Autodesk Inventor part; units mm, degrees
ref_plane "YZ Plane" through (0, 0, 0) normal (1, 0, 0) x (0, 1, 0)
ref_plane "XZ Plane" through (0, 0, 0) normal (0, 1, 0) x (-1, 0, 0)
ref_plane "XY Plane" through (0, 0, 0) normal (0, 0, 1) x (1, 0, 0)
sketch "スケッチ5" plane through (0, 0, 0) normal (1, 0, 0) x (0, 1, 0)
  line L0 (0, 0) -> (0, 1.2936) construction
  line L1 (0, 0) -> (-1.3338, 0) construction
  line L2 (2, 2) -> (-2, 2)
  line L3 (-2, 2) -> (-2, 0)
  line L4 (-2, 0) -> (2, 0)
  line L5 (2, 0) -> (2, 2)
  line L6 (0.8, 2) -> (0.8, 0)
  line L7 (-0.8, 2) -> (-0.8, 0)
  line L8 (-2, 1) -> (2, 1) construction
  line L9 (2, 1) -> (7.1642, 10.7124) construction
  line L10 (8.0471, 10.243) -> (6.2812, 11.1819)
  line L11 (6.2812, 11.1819) -> (0.7025, 0.6899)
  line L12 (0.7025, 0.6899) -> (2.4684, -0.2491)
  line L13 (2.4684, -0.2491) -> (8.0471, 10.243)
  line L14 (2, 0) -> (2.6009, 0)
  line L15 (6.6791, 14.0017) -> (4.7997, 13.3177)
  line L16 (4.7997, 13.3177) -> (6.1677, 9.5589)
  line L17 (6.1677, 9.5589) -> (8.0471, 10.243)
  line L18 (8.0471, 10.243) -> (6.6791, 14.0017)
  line L19 (6.6791, 14.0017) -> (6.1677, 9.5589) construction
  line L20 (4.7997, 13.3177) -> (8.0471, 10.243) construction
  line L21 (5.7394, 13.6597) -> (7.1074, 9.9009) construction
  line L22 (6.4234, 11.7803) -> (4.7515, 8.1465) construction
  line L23 (4.7515, 8.1465) -> (4.3748, 5.4664) construction
  line L24 (6.2812, 11.1819) -> (2.4684, -0.2491) construction
  line L25 (0.7025, 0.6899) -> (8.0471, 10.243) construction
  line L26 (7.3319, 11.3623) -> (5.5149, 12.1983)
  line L27 (5.5149, 12.1983) -> (3.843, 8.5645)
  line L28 (3.843, 8.5645) -> (5.66, 7.7285)
  line L29 (5.66, 7.7285) -> (7.3319, 11.3623)
  line L30 (7.3319, 11.3623) -> (3.843, 8.5645) construction
  line L31 (5.5149, 12.1983) -> (5.66, 7.7285) construction
  line L32 (5.66, 7.7285) -> (5.2826, 5.0437)
  line L33 (3.843, 8.5645) -> (2.6532, 0.0985)
  line L34 (3.467, 5.8892) -> (5.2329, 4.9502)
  point P0 (1.3991, 2)
  point P1 (5.5874, 9.9634)
  point P2 (5.3431, 11.8247)
  point P3 (6.5694, 9.7051)
  dimension "d25" = 1.6
  dimension "d26" = 4
  dimension "d27" = 2
  dimension "d28" = 118
  dimension "d29" = 2
  dimension "d30" = 11
  dimension "d44" = 2
  dimension "d45" = 20
  dimension "d46" = 4
  dimension "d52" = 20
  dimension "d53" = 4
  dimension "d54" = 2
extrude "押し出し8" add sketch "スケッチ5" along normal mid plane 3 contours L6 L11 L12 L4 L7 L2 | L2 L11 L6 | L7 L4 L3 L2 | L2 L5 L12 L6 L11 | L6 L12 L11 | L12 L4 L6
ref_plane "作業平面7" through (-1.5, -2, 2) normal (0, 0, 1) x (1, 0, 0)
sketch "スケッチ6" plane through (-1.5, -2, 2) normal (0, 0, 1) x (1, 0, 0)
  line L0 (3, 0) -> (0, 0)
  line L1 (3, 4) -> (3, 0)
  line L2 (0, 4) -> (3, 4)
  line L3 (0, 0) -> (0, 4)
  line L4 (0, 4) -> (3, 4)
  line L5 (0, 4) -> (3, 0) construction
  line L6 (0, 0) -> (3, 0)
  line L7 (3, 0) -> (3, 4)
  line L8 (0, 0) -> (3, 4) construction
  circle A0 centre (1.5, 2) radius 0.8
  dimension "d35" = 1.6
extrude "押し出し9" cut sketch "スケッチ6" against normal blind 4 contours A0
extrude "押し出し13" add sketch "スケッチ5" along normal blind 7 contours L16 L27 L26 L29 L10 L11 | L11 L10 L29 L17 L16 | L16 L15 L18 L10 L29 L26 L27 | L29 L10 L17
extrude "押し出し15" add sketch "スケッチ5" along normal mid plane 2 contours L11 L33 L13 L14 L5 L2 | L33 L28 L11 | L34 L13 L33 | L11 L28 L32 L13 L34 | L28 L27 L16 L11 | L11 L16 L17 L29 L28 | L16 L27 L26 L29 L10 L11 | L11 L10 L29 L17 L16
extrude "押し出し16" add sketch "スケッチ5" against normal blind 1 contours L16 L15 L18 L10 L29 L26 L27 | L29 L10 L17
fillet "フィレット1" radius 0.8 1 edges at (0, 1.3991, 2)
fillet "フィレット2" radius 1 1 edges at (0, 2.6009, 0)
fillet "フィレット3" radius 3 4 edges at (0, 5.2826, 5.0437) (0, 3.467, 5.8892) (0, 3.843, 8.5645) (0, 5.66, 7.7285)
fillet "フィレット4" radius 3 2 edges at (0, 5.3431, 11.8247) (0, 6.5694, 9.7051)
fillet "フィレット6" radius 0.8 1 edges at (-1, 7.3631, 12.1223)
ref_plane "作業平面8" through (-0.2, 5.7394, 13.6597) normal (0, 0.9396926, 0.3420201) x (1, 0, 0)
sketch "スケッチ8" plane through (-0.2, 5.7394, 13.6597) normal (0, 0.9396926, 0.3420201) x (1, 0, 0)
  point P0 (0.2, 10.8729)
fillet "フィレット11" radius 0.8 2 edges at (7, 5.7394, 13.6597) (7, 7.1074, 9.9009)
fillet "フィレット12" radius 0.8 4 edges at (1, 2, 1) (-1, 2, 1) (-1.5, -2, 1) (1.5, -2, 1)
fillet "フィレット13" radius 0.4 1 edges at (1, 5.5444, 11.2714)
properties part number "battery-stopper-1"
Can you work these out from the model? Positions are in its coordinate system, mm. Round coordinates to 2 decimals unless told otherwise and drop trailing zeros. Loops run counter-clockwise (first coordinate to the right, second up) from the corner with the lowest first, then second, coordinate; pieces in that order, holes last. Notation, with made-up numbers: (-12.75, 65.25) -> (43.25, 65.25) arc R15 ccw to (43.25, 90.25) -> close; hole circle Ø4 at (-11, 15). An arc over 180 degrees is marked (long way). Answer in a Markdown table with one row per item.
Item 1: Suppose I cut it at D-D, the plane x = 6.75. List the corners of the cut face in (y, z) for me, plus the area to 3 significant figures.
Answer block:
| item | result |
|---|---|
| outline | (4.87, 13.11) -> (6.09, 9.76) -> (7.97, 10.45) -> (6.75, 13.8) -> close |
| area | 7.12 mm² |
Item 2: Suppose I cut it at B-B, the plane x = 0. List the corners of the cut face in (y, z) for me.
Answer block:
| item | result |
|---|---|
| outline | (-2, 0) -> (-0.8, 0) -> (-0.8, 2) -> (-2, 2) -> close; (0.8, 0) -> (2, 0) arc R1 ccw to (2.88, 0.53) -> (5.03, 4.58) arc R3 ccw to (5.36, 5.57) -> (5.6, 7.29) arc R3 cw to (5.84, 8.13) -> (6.05, 8.57) arc R3 cw to (7.75, 10.13) -> (8.05, 10.24) -> (6.68, 14) -> (4.8, 13.32) -> (4.92, 12.98) arc R3 cw to (4.83, 10.7) -> (4.03, 8.96) arc R3 ccw to (3.78, 8.13) -> (3.54, 6.41) arc R3 cw to (3.22, 5.42) -> (1.62, 2.42) arc R0.8 cw to (0.92, 2) -> (0.8, 2) -> close |
Item 3: If I drill on probe 1 along Y at (x, z) = (0, 1.05); probe 2 along Y at (x, z) = (0.5, 1); probe 3 along X at (y, z) = (3.25, 3), over which ranges is the centre line in solid material (lowest first)?
Answer block:
| item | result |
|---|---|
| probe 1 | -2 to -0.8, 0.8 to 3.16 |
| probe 2 | -2 to -0.62, 0.62 to 3.13 |
| probe 3 | -1 to 1 |
Item 4: Suppose I cut it at C-C, the plane z = 3. List the corners of the cut face in (x, y) for me, plus the area to 3 significant figures.
Answer block:
| item | result |
|---|---|
| outline | (-1, 1.93) -> (1, 1.93) -> (1, 4.2) -> (-1, 4.2) -> close |
| area | 4.53 mm² |
Item 5: Will these pins go through, and if not, where does the flat tip stop? P1, Ø5, axis at x = 0, z = 4, coming from the +Y side; P2, Ø1, axis at y = 3, z = 3.5, coming from the -X side; P3, Ø1.5, axis at x = -0.5, y = 1.5, coming from the +Z side.
Answer block:
| item | result |
|---|---|
| P1 | y = 5.49 |
| P2 | x = -1 |
| P3 | z = 3.6 |
Item 6: Suppose I cut it at A-A, the plane y = 0. List the corners of the cut face in (x, z) for me, plus the area to 3 significant figures.
Answer block:
| item | result |
|---|---|
| outline | (-1.5, 0) -> (-0.8, 0) -> (-0.8, 2) -> (-1.5, 2) -> close; (0.8, 0) -> (1.5, 0) -> (1.5, 2) -> (0.8, 2) -> close |
| area | 2.80 mm² |
